Study the drawing (mm; zero at the part's minimum x, y, z) and answer. Coordinates: 2 decimals unless noted, no trailing zeros. Loops run counter-clockwise (first coordinate to the right, second up) from the corner with the lowest first, then second, coordinate; pieces in that order, holes last. Notation, with made-up numbers: (24, -3.75) - (60, -3.75) arc R11 ccw to (60, 17.25) - close; hole circle Ø2 at (-30, 20). An arc over 180 degrees is marked (long way). Put each result on its own line as item: value.
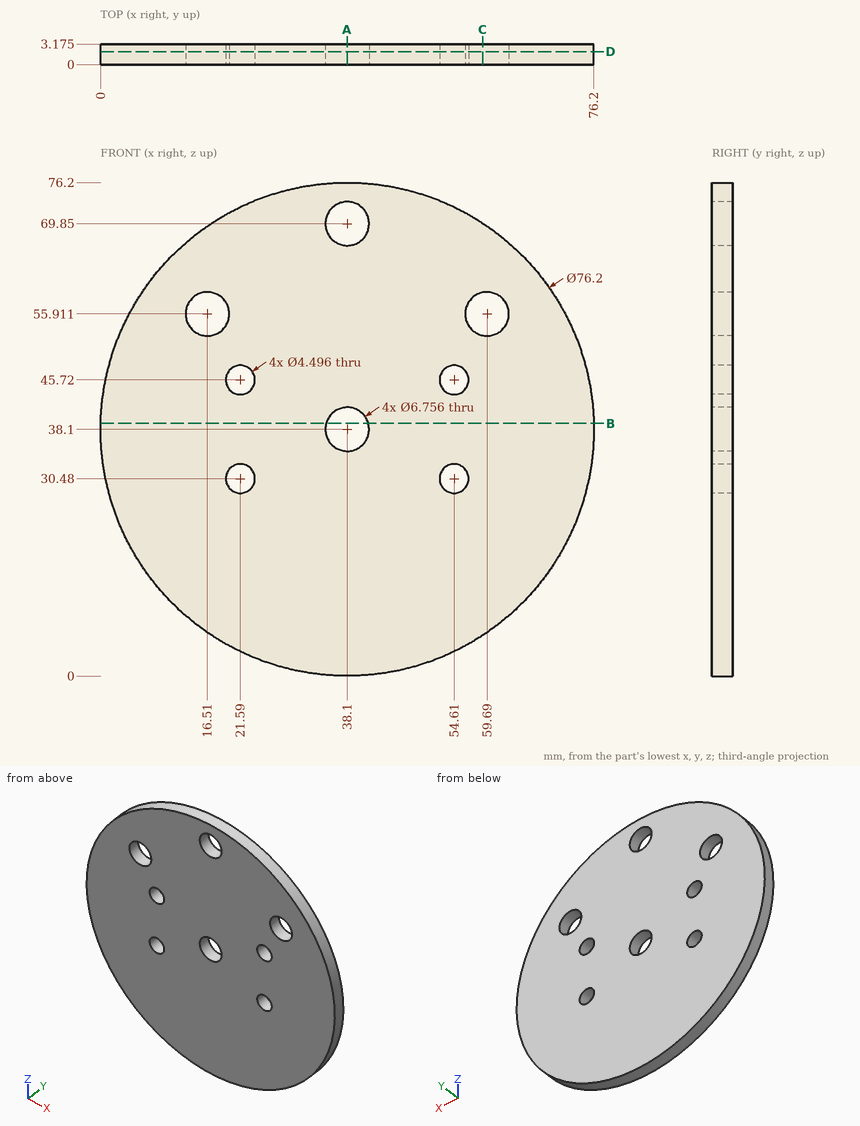
1) Straight lines are drawn through the part: L1, parallel to X at y = 1.65, z = 38.1; L2, parallel to Z at x = 54.61, y = 1.35; L3, parallel to Z at x = 23.5, y = 2.1 (1 decimal). For each, find the intervals that lie inside material, in ascending order. Write a range as [from, to].
Found:
L1: x = [0, 34.72], [41.48, 76.2]
L2: z = [3.76, 28.23], [32.73, 43.47], [47.97, 72.44]
L3: z = [2.9, 29.3], [31.7, 44.5], [46.9, 73.3]
2) The part is cut by section B-B (z = 39). Give the vertices of the cut face in (x, y) (1 decimal).
Found:
outline: (0, 0) - (34.8, 0) - (34.8, 3.2) - (0, 3.2) - close; (41.4, 0) - (76.2, 0) - (76.2, 3.2) - (41.4, 3.2) - close
3) Each of these flat-tipped pins is pushed along its axis until it touches: pin 1 (3.5 mm diameter, centred on x = 54.61, z = 45.72, fed in from +Y); pin 2 (1.5 mm diameter, centred on y = 1, z = 45.5, fed in from -X) (1 decimal). Where does it stop, or does it pass through?
Found:
pin 1: passes through
pin 2: stops at x = 0.6
4) The part is cut by section C-C (x = 59). Give the vertices of the cut face in (y, z) (1 decimal), and give its area (3 significant figures).
Found:
outline: (0, 6.2) - (3.2, 6.2) - (3.2, 52.6) - (0, 52.6) - close; (0, 59.2) - (3.2, 59.2) - (3.2, 70) - (0, 70) - close
area: 181 mm^2
5) The part is cut by section D-D (y = 2). State how many separate pieces and enclosed holes the cut face has, and give its area (3 significant figures).
Found:
separate pieces: 1
enclosed holes: 8
area: 4,350 mm^2
6) The part is cut by section A-A (x = 38.1). Give the vertices of the cut face in (y, z) (1 decimal).
Found:
outline: (0, 0) - (3.2, 0) - (3.2, 34.7) - (0, 34.7) - close; (0, 41.5) - (3.2, 41.5) - (3.2, 66.5) - (0, 66.5) - close; (0, 73.2) - (3.2, 73.2) - (3.2, 76.2) - (0, 76.2) - close
